Build history of the part. All positions in model axes, mm. A direction names the side the tool comes from. Give positions to 0.01 mm unless a question says otherwise; leave off trailing zeros. Write each loop counter-clockwise with the first axis right and the second up, starting at its lowest first coordinate (ties: lowest second). Pieces come first, ordered by that corner, then holes. Notation, with made-up numbers: M -28.75,-5.75 L 9.25,-5.75 A9 cw 9.25,3.25 Z; hole C -16.5,48 d11. An arc over 180 degrees is marked long. Return JSON: item names as keys, results as strings. Group by question number.
Q1. Tool access for faces 4 (the cylindrical face through (45.596, -27.756, 17.349)), 5 (the flat face through (-50, -20, 6.35)), 6 (the cylindrical face through (-50.984, -33.144, 16.097)): list every direction of +Z, -Z, +X, -X, +Y, -Y with a clear straight run to the whole face (end or side of a thin tool).
Q2. Band-saw the part on C-C, the plane x = -28.5. Give the cut face in (y, z), then the cut area to 3 significant figures.
Q3. Pull direction Y, two halves, no side cores. Call faces 1 (the flat face through (52.07, 0, 16)), 2 (the flat face through (48.26, 0, 17)), 3 (the flat face through (-1, -34.29, 16)): +Y half, -Y half, draft (parallel to the pull), parting line (faces both ways), or undercut.
Q4. Wall check: probe 1 along Y at (x, z) = (-48, 25); probe 2 along Y at (x, z) = (39, 26); probe 3 along X at (y, z) = (22, 25). Give the ranges that are in metal, low to high.
Q5. Band-saw the part on B-B, the plane z = 28. Count the separate pieces of the cut face and the enclosed holes in it, then the cut area to 3 significant figures.
Q6. Flat gauge pins, fed straight in: pin 1 Ø8 at (x, y) = (-40, 11.5) entering from +Z; pin 2 Ø0.9 at (x, y) = (48, -29.5) entering from +Z; pin 3 Ø1.1 at (x, z) = (-50.5, 11.5) entering from +Y. Where does each tip first touch, or does it go through?
Q7. Band-saw the part on A-A, the plane y = -18. Give the cut face in (x, z).
from build123d import *

# Parameters (mm, degrees)
F0_W     = 104.14
F0_H     = 68.58
F1_DEPTH = 31.75
F2_DEPTH = 12.7
F3_DEPTH = 2.54
F4_W     = 12.7
F4_H     = 12.7
F4_W_2   = 11.43
F4_H_2   = 20.32
F5_DEPTH = 10.16
F6_R     = 3.81
F7_R     = 3.80999
F8_DEPTH = 12.7


# Not quite as in the source:
# - a fillet or chamfer is up to 0.001 mm smaller than in the source, because OpenCascade refuses the exact size


with BuildPart() as f1:
    # F0 (on Top) → F1 (new body)
    with BuildSketch(Plane.XY):
        Rectangle(F0_W, F0_H)
        with BuildLine():
            ThreePointArc((-48.26, 28.956), (-49.3376307345, 31.5576307345), (-46.736, 30.48))
            Line((-46.736, 30.48), (-44.45, 30.48))
            Line((-44.45, 30.48), (22.86, 30.48))
            Line((22.86, 30.48), (25.4, 30.48))
            Line((25.4, 30.48), (44.45, 30.48))
            Line((44.45, 30.48), (46.736, 30.48))
            ThreePointArc((46.736, 30.48), (48.26, 32.004), (49.784, 30.48))
            ThreePointArc((49.784, 30.48), (49.3376307345, 29.4023692655), (48.26, 28.956))
            Line((48.26, 28.956), (48.26, 26.67))
            Line((48.26, 26.67), (48.26, -26.67))
            Line((48.26, -26.67), (48.26, -28.956))
            ThreePointArc((48.26, -28.956), (49.3376307345, -29.4023692655), (49.784, -30.48))
            ThreePointArc((49.784, -30.48), (48.26, -32.004), (46.736, -30.48))
            Line((46.736, -30.48), (44.45, -30.48))
            Line((44.45, -30.48), (25.4, -30.48))
            Line((25.4, -30.48), (22.86, -30.48))
            Line((22.86, -30.48), (-44.45, -30.48))
            Line((-44.45, -30.48), (-46.736, -30.48))
            ThreePointArc((-46.736, -30.48), (-49.3376307345, -31.5576307345), (-48.26, -28.956))
            Line((-48.26, -28.956), (-48.26, -26.67))
            Line((-48.26, -26.67), (-48.26, 26.67))
            Line((-48.26, 26.67), (-48.26, 28.956))
        make_face(mode=Mode.SUBTRACT)
        with BuildLine():
            Line((46.736, 30.48), (44.45, 30.48))
            Line((44.45, 30.48), (44.45, 26.67))
            Line((44.45, 26.67), (48.26, 26.67))
            Line((48.26, 26.67), (48.26, 28.956))
            ThreePointArc((48.26, 28.956), (47.1823692655, 29.4023692655), (46.736, 30.48))
        make_face()
        with BuildLine():
            Line((48.26, -28.956), (48.26, -26.67))
            Line((48.26, -26.67), (44.45, -26.67))
            Line((44.45, -26.67), (44.45, -30.48))
            Line((44.45, -30.48), (46.736, -30.48))
            ThreePointArc((46.736, -30.48), (47.1823692655, -29.4023692655), (48.26, -28.956))
        make_face()
        with BuildLine():
            Line((-44.45, -26.67), (-48.26, -26.67))
            Line((-48.26, -26.67), (-48.26, -28.956))
            ThreePointArc((-48.26, -28.956), (-47.1823692655, -29.4023692655), (-46.736, -30.48))
            Line((-46.736, -30.48), (-44.45, -30.48))
            Line((-44.45, -30.48), (-44.45, -26.67))
        make_face()
        with BuildLine():
            Line((-44.45, 30.48), (-46.736, 30.48))
            ThreePointArc((-46.736, 30.48), (-47.1823692655, 29.4023692655), (-48.26, 28.956))
            Line((-48.26, 28.956), (-48.26, 26.67))
            Line((-48.26, 26.67), (-44.45, 26.67))
            Line((-44.45, 26.67), (-44.45, 30.48))
        make_face()
    extrude(amount=F1_DEPTH)

    # F0 (on Top) → F2 (join)
    with BuildSketch(Plane.XY):
        Polygon((25.4, 30.48), (22.86, 30.48), (22.86, 19.05), (26.67, 15.24), (26.67, -24.13), (22.86, -27.94), (22.86, -30.48), (25.4, -30.48), (25.4, -27.94), (29.21, -24.13), (29.21, 15.24), (25.4, 19.05), align=None)
    extrude(amount=F2_DEPTH)

    # F0 (on Top) → F3 (join)
    with BuildSketch(Plane.XY):
        Polygon((22.86, 30.48), (-44.45, 30.48), (-44.45, 26.67), (-48.26, 26.67), (-48.26, -26.67), (-44.45, -26.67), (-44.45, -30.48), (22.86, -30.48), (22.86, -27.94), (26.67, -24.13), (26.67, 15.24), (22.86, 19.05), align=None)
        Polygon((44.45, 30.48), (25.4, 30.48), (25.4, 19.05), (29.21, 15.24), (29.21, -24.13), (25.4, -27.94), (25.4, -30.48), (44.45, -30.48), (44.45, -26.67), (48.26, -26.67), (48.26, 26.67), (44.45, 26.67), align=None)
    extrude(amount=F3_DEPTH)

    # F4 (on face) → F5 (cut)
    with BuildSketch(Plane(origin=(-52.07, 0, 0), x_dir=(0, -1, 0), z_dir=(-1, 0, 0))):
        with Locations((-11.43, 12.7)):
            Rectangle(F4_W, F4_H)
        with Locations((19.685, 16.51)):
            Rectangle(F4_W_2, F4_H_2)
    extrude(amount=-F5_DEPTH, mode=Mode.SUBTRACT)

    # F6
    f6_edges = [f1.edges().sort_by_distance(p)[0] for p in [
        (-52.07, -34.29, 15.875),
        (52.07, -34.29, 15.875),
        (52.07, 34.29, 15.875),
        (-52.07, 34.29, 15.875),
    ]]
    fillet(f6_edges, radius=F6_R)

    # F7 (radius 3.81 in the source; OpenCascade refuses exactly that, so slightly less here)
    f7_edges = [f1.edges().sort_by_distance(p)[0] for p in [
        (44.45, 26.67, 17.145),
        (-44.45, 26.67, 17.145),
        (44.45, -26.67, 17.145),
        (-44.45, -26.67, 17.145),
    ]]
    fillet(f7_edges, radius=F7_R)

    # F0 (on Top) → F8 (join)
    with BuildSketch(Plane.XY):
        with BuildLine():
            Line((-48.26, 28.956), (-48.26, 30.48))
            Line((-48.26, 30.48), (-46.736, 30.48))
            ThreePointArc((-46.736, 30.48), (-49.3376307345, 31.5576307345), (-48.26, 28.956))
        make_face()
        with BuildLine():
            Line((48.26, 30.48), (46.736, 30.48))
            ThreePointArc((46.736, 30.48), (47.1823692655, 29.4023692655), (48.26, 28.956))
            Line((48.26, 28.956), (48.26, 30.48))
        make_face()
        with BuildLine():
            ThreePointArc((49.784, 30.48), (48.26, 32.004), (46.736, 30.48))
            Line((46.736, 30.48), (48.26, 30.48))
            Line((48.26, 30.48), (48.26, 28.956))
            ThreePointArc((48.26, 28.956), (49.3376307345, 29.4023692655), (49.784, 30.48))
        make_face()
        with BuildLine():
            Line((-46.736, 30.48), (-48.26, 30.48))
            Line((-48.26, 30.48), (-48.26, 28.956))
            ThreePointArc((-48.26, 28.956), (-47.1823692655, 29.4023692655), (-46.736, 30.48))
        make_face()
        with BuildLine():
            Line((-48.26, -30.48), (-48.26, -28.956))
            ThreePointArc((-48.26, -28.956), (-49.3376307345, -31.5576307345), (-46.736, -30.48))
            Line((-46.736, -30.48), (-48.26, -30.48))
        make_face()
        with BuildLine():
            ThreePointArc((-46.736, -30.48), (-47.1823692655, -29.4023692655), (-48.26, -28.956))
            Line((-48.26, -28.956), (-48.26, -30.48))
            Line((-48.26, -30.48), (-46.736, -30.48))
        make_face()
        with BuildLine():
            ThreePointArc((49.784, -30.48), (49.3376307345, -29.4023692655), (48.26, -28.956))
            Line((48.26, -28.956), (48.26, -30.48))
            Line((48.26, -30.48), (46.736, -30.48))
            ThreePointArc((46.736, -30.48), (48.26, -32.004), (49.784, -30.48))
        make_face()
        with BuildLine():
            Line((48.26, -30.48), (48.26, -28.956))
            ThreePointArc((48.26, -28.956), (47.1823692655, -29.4023692655), (46.736, -30.48))
            Line((46.736, -30.48), (48.26, -30.48))
        make_face()
    extrude(amount=F8_DEPTH)


solid = f1.part
From the geometry:
{
 "1": {"face 4": "+Z", "face 5": "-X", "face 6": "+Z, -Z, -X, -Y"},
 "2": {"outline": "M -34.29,0 L 34.29,0 L 34.29,31.75 L 30.48,31.75 L 30.48,2.54 L -30.48,2.54 L -30.48,31.75 L -34.29,31.75 Z", "area": "397 mm^2"},
 "3": {"face 1": "draft", "face 2": "undercut", "face 3": "-Y half"},
 "4": {"probe 1": "y = -34.29 to -31.98, -28.98 to -26.68, 26.68 to 28.98, 31.98 to 34.29", "probe 2": "y = -34.29 to -30.48, 30.48 to 34.29", "probe 3": "x = -52.07 to -48.26, 48.26 to 52.07"},
 "5": {"separate pieces": "1", "enclosed holes": "5", "area": "1,260 mm^2"},
 "6": {"pin 1": "stops at z = 2.54", "pin 2": "stops at z = 12.7", "pin 3": "stops at y = 33.89"},
 "7": {"outline": "M -52.07,0 L 52.07,0 L 52.07,31.75 L 48.26,31.75 L 48.26,2.54 L 29.21,2.54 L 29.21,12.7 L 26.67,12.7 L 26.67,2.54 L -48.26,2.54 L -48.26,6.35 L -52.07,6.35 Z; M -52.07,26.67 L -48.26,26.67 L -48.26,31.75 L -52.07,31.75 Z"}
}
